```python
from build123d import *

# Parameters (mm, degrees)
SKETCH1_R           = 21.5
SKETCH1_R_2         = 1.6
BOSS_EXTRUDE1_DEPTH = 2
FILLET1_R           = 10


with BuildPart() as part:
    # Sketch1 → Boss-Extrude1 (new body)
    with BuildSketch(Plane(origin=(0, 0, 0), x_dir=(1, 0, 0), z_dir=(0, 1, 0))):
        with BuildLine():
            Line((4, 26.196373795), (4, 64.5))
            ThreePointArc((4, 64.5), (0, 68.5), (-4, 64.5))
            Line((-4, 64.5), (-4, 26.196373795))
            ThreePointArc((-4, 26.196373795), (-18.738329701, 18.738329701), (-26.196373795, 4))
            Line((-26.196373795, 4), (-64.5, 4))
            ThreePointArc((-64.5, 4), (-68.5, 0), (-64.5, -4))
            Line((-64.5, -4), (-26.196373795, -4))
            ThreePointArc((-26.196373795, -4), (-18.738329701, -18.738329701), (-4, -26.196373795))
            Line((-4, -26.196373795), (-4, -64.5))
            ThreePointArc((-4, -64.5), (0, -68.5), (4, -64.5))
            Line((4, -64.5), (4, -26.196373795))
            ThreePointArc((4, -26.196373795), (18.738329701, -18.738329701), (26.196373795, -4))
            Line((26.196373795, -4), (64.5, -4))
            ThreePointArc((64.5, -4), (68.5, 0), (64.5, 4))
            Line((64.5, 4), (26.196373795, 4))
            ThreePointArc((26.196373795, 4), (18.738329701, 18.738329701), (4, 26.196373795))
        make_face()
        with Locations(Location((0, 0, 0), (0, 0, 270))):
            Circle(SKETCH1_R, mode=Mode.SUBTRACT)
        with Locations(Location((0, 64.5, 0), (0, 0, 270))):
            Circle(SKETCH1_R_2, mode=Mode.SUBTRACT)
        with Locations(Location((64.5, 0, 0), (0, 0, 270))):
            Circle(SKETCH1_R_2, mode=Mode.SUBTRACT)
        with Locations(Location((0, -64.5, 0), (0, 0, 270))):
            Circle(SKETCH1_R_2, mode=Mode.SUBTRACT)
        with Locations(Location((-64.5, 0, 0), (0, 0, 270))):
            Circle(SKETCH1_R_2, mode=Mode.SUBTRACT)
    extrude(amount=BOSS_EXTRUDE1_DEPTH)

    # Fillet1
    fillet1_edges = [part.edges().sort_by_distance(p)[0] for p in [
        (26.196373795, 1, -4),
        (26.196373795, 1, 4),
        (4, 1, 26.196373795),
        (-4, 1, 26.196373795),
        (-26.196373795, 1, 4),
        (-26.196373795, 1, -4),
        (-4, 1, -26.196373795),
        (4, 1, -26.196373795),
    ]]
    fillet(fillet1_edges, radius=FILLET1_R)


solid = part.part
```
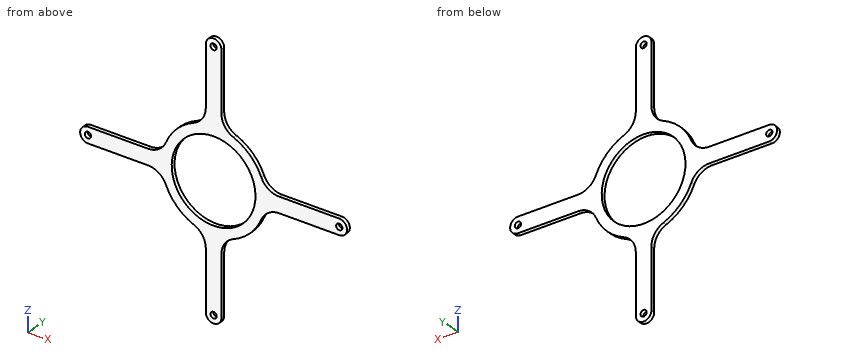
The model under review builds one solid part; all positions refer to its coordinate system, in mm. Round coordinates to 2 decimals unless told otherwise and drop trailing zeros. Loops run counter-clockwise (first coordinate to the right, second up) from the corner with the lowest first, then second, coordinate; pieces in that order, holes last.
1) Clearance check with flat-ended pins moving along their axes: P1, Ø1, axis at x = -49.5, y = 1.5, coming from the -Z side; P2, Ø0.6, axis at y = 1.5, z = 51.5, coming from the -X side; P3, Ø0.6, axis at y = 1.5, z = 55.5, coming from the +X side. State where each tip first meets the part, or that it passes through.
Values follow:
P1: stops at z = -4
P2: stops at x = -4
P3: stops at x = 4
2) Consider section A-A on x = 0. State the section outline as (y, z) points.
Values follow:
outline: (0, -68.5) - (2, -68.5) - (2, -66.1) - (0, -66.1) - close; (0, -62.9) - (2, -62.9) - (2, -21.5) - (0, -21.5) - close; (0, 21.5) - (2, 21.5) - (2, 62.9) - (0, 62.9) - close; (0, 66.1) - (2, 66.1) - (2, 68.5) - (0, 68.5) - close
3) Consider section C-C on y = 1.3. Give the number of separate pieces and of enclosed holes in the cut face, then the cut area to 3 significant figures.
Values follow:
separate pieces: 1
enclosed holes: 5
area: 2,120 mm2
4) Consider section D-D on x = 16. State the section outline as (y, z) points, then the cut area to 3 significant figures.
Values follow:
outline: (0, -21.12) - (2, -21.12) - (2, -14.36) - (0, -14.36) - close; (0, 14.36) - (2, 14.36) - (2, 21.12) - (0, 21.12) - close
area: 27.1 mm2
5) Wall thickness on line 1 along X through (y, z) = (1.45, 0); line 2 along X through (y, z) = (1.55, 64.5): over which ranges is each line inside the solid? List them lowest first.
Values follow:
line 1: x = -68.5 to -66.1, -62.9 to -21.5, 21.5 to 62.9, 66.1 to 68.5
line 2: x = -4 to -1.6, 1.6 to 4
6) Consider section B-B on z = 0. State the section outline as (x, y) points.
Values follow:
outline: (-68.5, 0) - (-66.1, 0) - (-66.1, 2) - (-68.5, 2) - close; (-62.9, 0) - (-21.5, 0) - (-21.5, 2) - (-62.9, 2) - close; (21.5, 0) - (62.9, 0) - (62.9, 2) - (21.5, 2) - close; (66.1, 0) - (68.5, 0) - (68.5, 2) - (66.1, 2) - close
